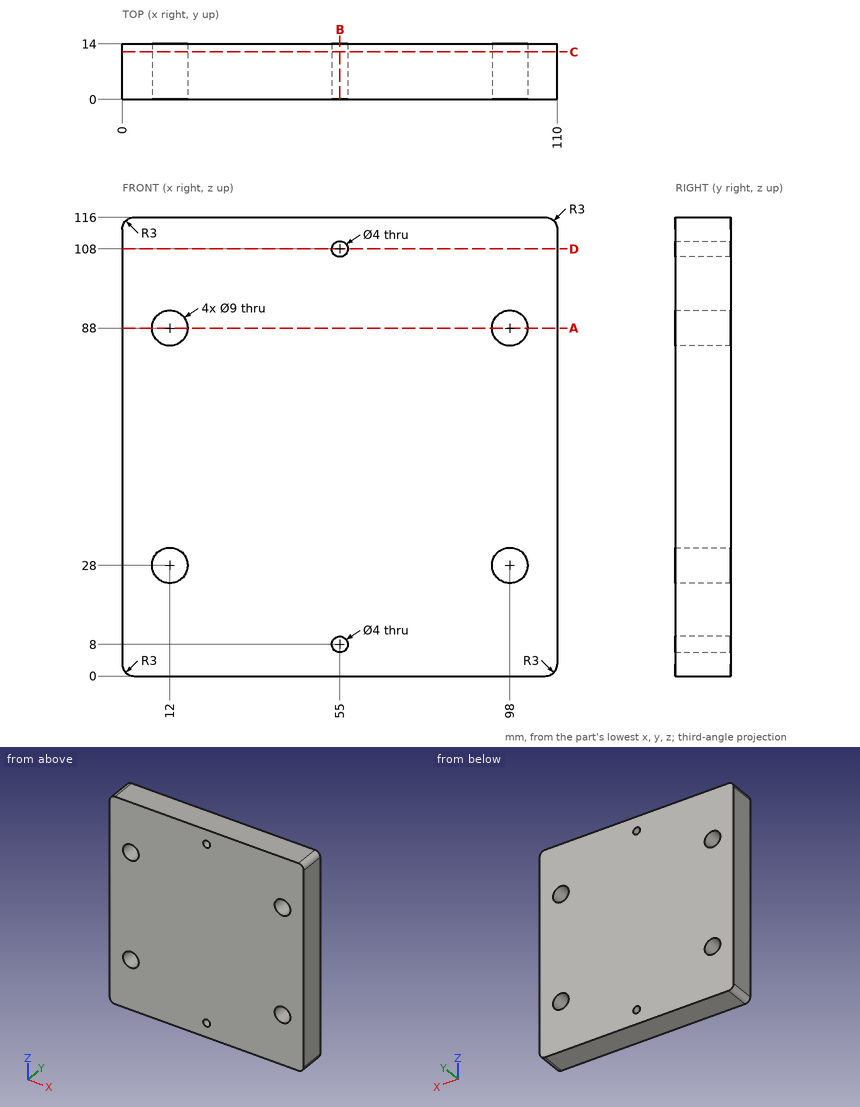
Here's the drawing with two shaded views (mm, measured from the low corner). I have some questions. Coordinates: 2 decimals unless noted, no trailing zeros. Write each loop counter-clockwise with the first axis right and the second up, starting at its lowest first coordinate (ties: lowest second). Pieces come first, ordered by that corner, then holes. Notation, with made-up numbers: M -8.5,38 L 26.5,38 A15 ccw 26.5,43 Z; hole C -6.5,-4 d8. An arc over 180 degrees is marked long. Write item = value, one per line. Start each with the question number.
Q1. If we section it at C-C, the plane y = 12: Write out the boundary of the cut face in (x, z).
Q2. I'm going to push a flat-ended pin straight in: pin 1 (10.5 mm diameter, centred on x = 12, z = 28, fed in from +Y). Where does the tip first touch, or does it pass through?
Q3. If I drill on L1, parallel to X at y = 10.5, z = 88; L2, parallel to Z at x = 94, y = 1.5; L3, parallel to Z at x = 56, y = 6.75, over which ranges is the centre line in solid material (lowest first)? Write a range as [from, to].
Q4. If we section it at D-D, the plane z = 108: Write out the boundary of the cut face in (x, y).
Q5. If we section it at A-A, the plane z = 88: Write out the boundary of the cut face in (x, y), then the cut area to 3 significant figures.
Q6. If we section it at B-B, the plane x = 55: Write out the boundary of the cut face in (y, z).
Check sheet entries:
q1.outline = M 0,3 A3 ccw 3,0 L 107,0 A3 ccw 110,3 L 110,113 A3 ccw 107,116 L 3,116 A3 ccw 0,113 Z; hole C 12,28 d9; hole C 12,88 d9; hole C 55,8 d4; hole C 55,108 d4; hole C 98,28 d9; hole C 98,88 d9
q2.pin_1 = 14
q3.L1 = [0, 7.5], [16.5, 93.5], [102.5, 110]
q3.L2 = [0, 25.94], [30.06, 85.94], [90.06, 116]
q3.L3 = [0, 6.27], [9.73, 106.27], [109.73, 116]
q4.outline = M 0,0 L 53,0 L 53,14 L 0,14 Z; M 57,0 L 110,0 L 110,14 L 57,14 Z
q5.outline = M 0,0 L 7.5,0 L 7.5,14 L 0,14 Z; M 16.5,0 L 93.5,0 L 93.5,14 L 16.5,14 Z; M 102.5,0 L 110,0 L 110,14 L 102.5,14 Z
q5.area = 1,290 mm²
q6.outline = M 0,0 L 14,0 L 14,6 L 0,6 Z; M 0,10 L 14,10 L 14,106 L 0,106 Z; M 0,110 L 14,110 L 14,116 L 0,116 Z
